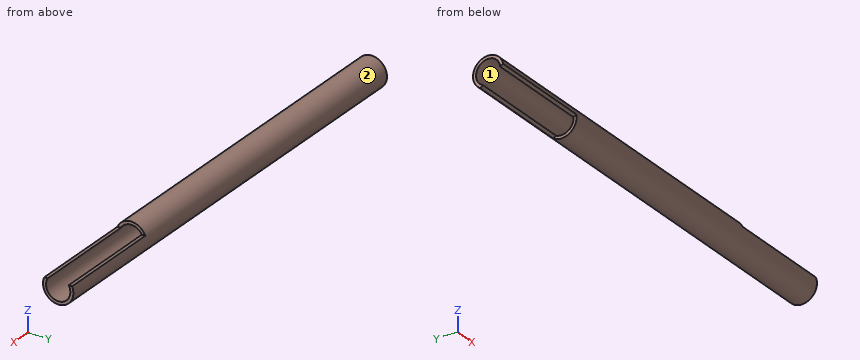
```python
from build123d import *

# Parameters (mm, degrees)
F0_R     = 5
F0_R_2   = 4
F1_DEPTH = 150
F3_DEPTH = 5
F5_W     = 35
F5_H     = 10
F6_DEPTH = 12.5


with BuildPart() as f1:
    # F0 (on Right) → F1 (new body)
    with BuildSketch(Plane.YZ):
        Circle(F0_R)
        Circle(F0_R_2, mode=Mode.SUBTRACT)
    extrude(amount=F1_DEPTH)

    # F2 (on Front) → F3 (cut, symmetric)
    with BuildSketch(Plane.XZ):
        Polygon((115, 2), (150, 2), (150, 5), (150, 12), (115, 12), align=None)
    extrude(amount=F3_DEPTH, both=True, mode=Mode.SUBTRACT)

    # F5 (on face) → F6 (cut, symmetric)
    with BuildSketch(Plane(origin=(0, 0, 0), x_dir=(1, 0, 0), z_dir=(0, -0.821816, 0.569753))):
        with Locations((17.5, -7)):
            Rectangle(F5_W, F5_H)
    extrude(amount=F6_DEPTH, both=True, mode=Mode.SUBTRACT)


solid = f1.part
```
Geometry: final body of the model. Coordinates: model frame, mm. Face numbers are marked on the shaded views. Coordinates: 2 decimals unless noted, no trailing zeros. Loops run counter-clockwise (first coordinate to the right, second up) from the corner with the lowest first, then second, coordinate; pieces in that order, holes last. Notation, with made-up numbers: (-18, -35.75) -> (-12, -35.75) arc R23 cw to (-12, -22.75) -> close; hole circle Ø3 at (-21, 13). An arc over 180 degrees is marked (long way). Use a Markdown table: item, result. Add a question column.
(1) Line query: line 1 along Y through (x, z) = (94.5, 0); line 2 along Z through (x, y) = (73, -2). Output: solid intervals per line, ascending.
(2) Pin query (flat end, axial travel): pin 1 Ø2 at (x, y) = (118.5, 4) entering from -Z; pin 2 Ø4 at (y, z) = (1, 2) entering from +X; pin 3 Ø1 at (x, y) = (101.5, -2.5) entering from +Z; pin 4 Ø3 at (y, z) = (-1, 1) entering from -X. Return the tip coordinate at first contact, or that it passes through.
(3) Section query B-B, the plane z = -1.25. Return loops of the section in (x, y), plus the area to 3 significant figures.
(4) Section query D-D, the plane x = 30. Return loops of the section in (y, z), plus the area to 3 significant figures.
(5) Mould query, pull axis Z, two halves, no side actions, for the marked faces 1 and 2. Classes: pulls with the +Z half, pulls with the -Z half, needs draft (parallel to the pull), parting line crosses it, or undercut.
(6) Section query A-A, the plane y = 0. Return loops of the section in (x, z).
(7) Section query C-C, the plane x = 49.5. Return loops of the section in (y, z).
Answer:
| question | item | result |
|---|---|---|
| 1 | line 1 | y = -5 to -4, 4 to 5 |
| 1 | line 2 | z = -4.58 to -3.46, 3.46 to 4.58 |
| 2 | pin 1 | stops at z = -4 |
| 2 | pin 2 | stops at x = 115 |
| 2 | pin 3 | stops at z = 4.58 |
| 2 | pin 4 | passes through |
| 3 | outline | (0, 3.8) -> (150, 3.8) -> (150, 4.84) -> (0, 4.84) -> close; (35, -4.84) -> (150, -4.84) -> (150, -3.8) -> (35, -3.8) -> close |
| 3 | area | 276 mm^2 |
| 4 | outline | (-4.91, 0.97) -> (-3.99, 0.33) arc R4 cw (long way) to (1.71, -3.62) -> (2.63, -4.25) arc R5 ccw (long way) to start |
| 4 | area | 18.3 mm^2 |
| 5 | face 1 | undercut |
| 5 | face 2 | parting line crosses it |
| 6 | outline | (0, 4) -> (115, 4) -> (115, 5) -> (0, 5) -> close; (35, -5) -> (150, -5) -> (150, -4) -> (35, -4) -> close |
| 7 | outline | circle Ø10 at (0, 0); hole circle Ø8 at (0, 0) |
